The listing builds one solid part. Answer for the finished solid, in the listing's coordinates (mm). A direction names the side the tool comes from. Give positions to 0.01 mm unless a question says otherwise; leave off trailing zeros. Order: outer loops, then holes, each group sorted by start corner. A loop starts at its lowest first (then second) coordinate and runs counter-clockwise, first axis right, second up.
Autodesk Inventor part; units mm, degrees
ref_plane "YZ Plane" through (0, 0, 0) normal (1, 0, 0) x (0, 1, 0)
ref_plane "XZ Plane" through (0, 0, 0) normal (0, 1, 0) x (-1, 0, 0)
ref_plane "XY Plane" through (0, 0, 0) normal (0, 0, 1) x (1, 0, 0)
sketch "Sketch1" plane through (0, 0, 0) normal (0, 0, 1) x (1, 0, 0)
  line L0 (0, 0) -> (50.8, 0)
  line L1 (50.8, 0) -> (50.8, 76.2)
  line L2 (50.8, 76.2) -> (0, 76.2)
  line L3 (0, 76.2) -> (0, 0)
  dimension "d0" = 50.8
  dimension "d1" = 76.2
extrude "Extrusion1" add sketch "Sketch1" along normal blind 6.35
sketch "Sketch2" plane through (0, 0, 0) normal (0, -1, 0) x (1, 0, 0)
  line L0 (0, 0) -> (50.8, 0)
  line L1 (0, 6.35) -> (50.8, 6.35)
  line L2 (0, 0) -> (50.8, 0)
  line L3 (50.8, 0) -> (50.8, 6.35)
  line L4 (50.8, 6.35) -> (0, 6.35)
  line L5 (0, 6.35) -> (0, 0)
  line L6 (49.2125, 4.7625) -> (49.2125, 1.5875)
  line L7 (49.2125, 1.5875) -> (1.5875, 1.5875)
  line L8 (1.5875, 1.5875) -> (1.5875, 4.7625)
  line L9 (1.5875, 4.7625) -> (49.2125, 4.7625)
  dimension "d4" = 1.5875
extrude "Extrusion2" cut sketch "Sketch2" against normal blind 63.5 contours L6 L7 L8 L9
sketch "Sketch3" plane through (0, 0, 6.35) normal (0, 0, 1) x (1, 0, 0)
  line L0 (50.8, 76.2) -> (0, 76.2)
  line L1 (25.4, 76.2) -> (25.4, 0)
  line L2 (49.2125, 0) -> (1.5875, 0)
  line L3 (30.48, 76.2) -> (30.48, 0)
  line L4 (20.32, 76.2) -> (20.32, 0)
  line L5 (49.2125, 63.5) -> (1.5875, 63.5)
  line L6 (25.4, 63.5) -> (25.4, 50.8)
  line L7 (25.4, 50.8) -> (25.4, 45.72)
  circle A0 centre (25.4, 45.72) radius 5.08
  line L8 (30.48, 45.72) -> (30.48, 20.32)
  line L9 (49.2125, 0) -> (49.2125, 63.5)
  line L10 (30.48, 20.32) -> (49.2125, 0)
  line L11 (20.32, 45.72) -> (20.32, 20.32)
  line L12 (20.32, 20.32) -> (1.5875, 0)
  point P0 (0, 0)
  dimension "d7" = 5.08
  dimension "d8" = 5.08
  dimension "d9" = 12.7
  dimension "d10" = 5.08
  dimension "d11" = 25.4
  dimension "d12" = 25.4
extrude "Extrusion3" cut sketch "Sketch3" against normal blind 4.7625 contours A0 L1 | L3 L2 L1 A0 | L1 A0 | L10 L2 L3 | L1 L2 L4 A0 | L4 L2 L12
1) Straight lines are drawn through the part: probe 1 along X at (y, z) = (45, 2.5); probe 2 along Z at (x, y) = (39.5, 51.5); probe 3 along Y at (x, z) = (29, 3.5). For each, find the intervals that lie inside material, in ascending order.
Geometry says:
probe 1: x = 0 to 1.59, 49.21 to 50.8
probe 2: z = 0 to 1.59, 4.76 to 6.35
probe 3: y = 63.5 to 76.2
2) Find section C-C (x = 25.4). Write down the section's boundary in (y, z), then the cut area to 3 significant figures.
Geometry says:
outline: (0, 0) - (76.2, 0) - (76.2, 6.35) - (50.8, 6.35) - (50.8, 4.76) - (63.5, 4.76) - (63.5, 1.59) - (0, 1.59) - close
area: 202 mm2
3) Find section A-A (z = 3). Write down the section's boundary in (x, y).
Geometry says:
outline: (0, 0) - (1.59, 0) - (1.59, 63.5) - (49.21, 63.5) - (49.21, 0) - (50.8, 0) - (50.8, 76.2) - (0, 76.2) - close
4) Given P1, Ø1, axis at x = 30.5, z = 3.5, coming from the -Y side; P2, Ø3, axis at x = 23.5, z = 3.5, coming from the -Y side, each flat-ended and moving along its own axis, determine where each tip first touches the part or whether it passes through.
Geometry says:
P1: stops at y = 63.5
P2: stops at y = 50.02
5) A tool of negligible diameter and unlimited length cuts with its end or side. For faces 5 (the flat face through (25, 0, 1)), 6 (the flat face through (49.212, 31, 3)), 7 (the flat face through (30.48, 33, 6)), from which of +Z, -Z, +X, -X, +Y, -Y can it reach the whole face along a straight path? Write none if from no direction.
Geometry says:
face 5: +Z, -Z, +X, -X, -Y
face 6: -Y
face 7: +Z, -Y
6) Find section B-B (y = 24). Write down the section's boundary in (x, z), then the cut area to 3 significant figures.
Geometry says:
outline: (0, 0) - (50.8, 0) - (50.8, 6.35) - (30.48, 6.35) - (30.48, 4.76) - (49.21, 4.76) - (49.21, 1.59) - (1.59, 1.59) - (1.59, 4.76) - (20.32, 4.76) - (20.32, 6.35) - (0, 6.35) - close
area: 155 mm2
7) For a pull along Z with two mould halves and no side action, classify faces 1 (the flat face through (11.085, 10.302, 5.567)), 2 (the flat face through (1.588, 31, 3)), 3 (the flat face through (25, 39, 0)), 4 (the flat face through (19, 47, 6.35)) as +Z half, -Z half, draft (parallel to the pull), parting line (faces both ways), or undercut.
Geometry says:
face 1: draft
face 2: undercut
face 3: -Z half
face 4: +Z half
